Part print with two shaded views. Sizes in mm from the minimum x, y, z corner. A direction names the side the tool comes from. Give positions to 0.01 mm unless a question says otherwise; leave off trailing zeros. Order: outer loops, then holes, each group sorted by start corner. A loop starts at its lowest first (then second) coordinate and runs counter-clockwise, first axis right, second up. Notation, with made-up numbers: M 85.5,62.5 L 99.5,62.5 A26 ccw 99.5,99.5 Z; hole C 14.5,77 d11. An arc over 180 degrees is marked long. Return JSON: item names as keys, results as strings.
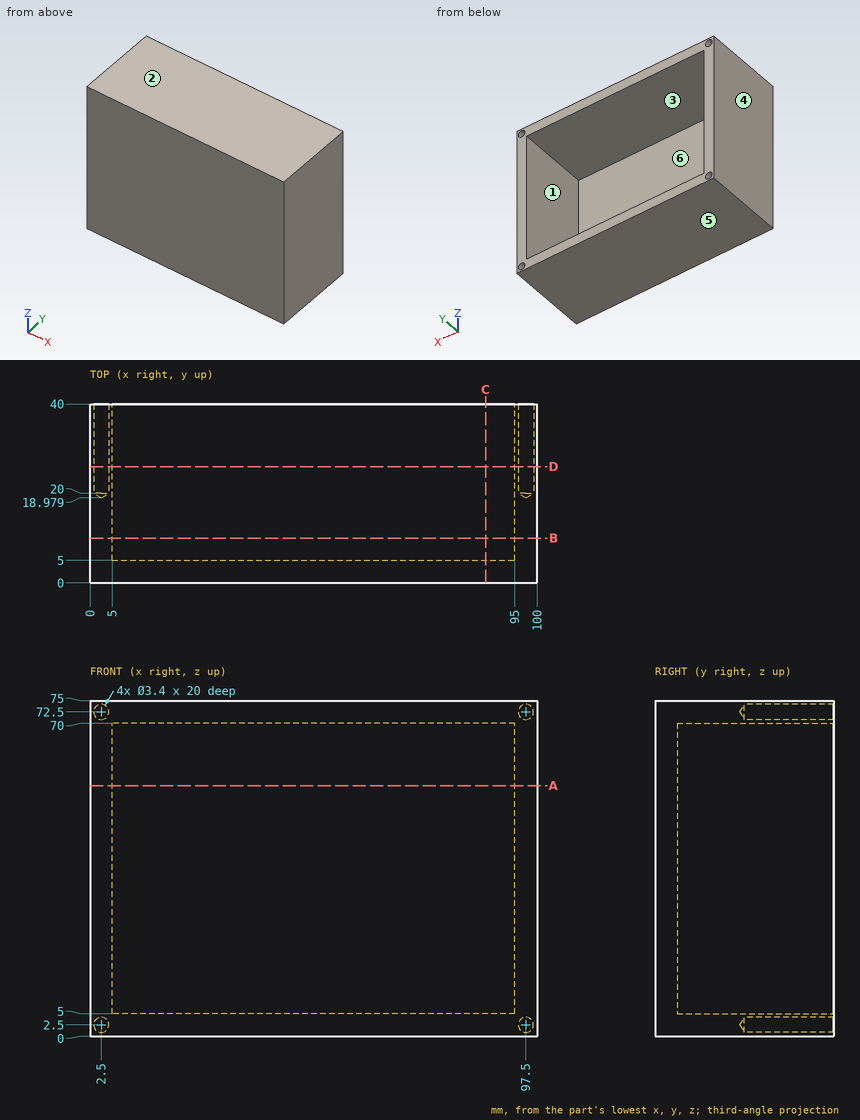
Q1. Two-plate mould, pull along Z, no slides. Class the marked faces 3, 4, 5 and 6: +Z half, -Z half, draft (parallel to the pull), parting line (faces both ways), or undercut.
Established:
{"face 3": "undercut", "face 4": "draft", "face 5": "-Z half", "face 6": "undercut"}
Q2. Band-saw the part on D-D (y = 26). Give the cut face in (x, z), then the cut area to 3 significant figures.
Established:
{"outline": "M 0,0 L 100,0 L 100,75 L 0,75 Z; hole C 2.5,2.5 d3.4; hole C 2.5,72.5 d3.4; hole M 5,5 L 95,5 L 95,70 L 5,70 Z; hole C 97.5,2.5 d3.4; hole C 97.5,72.5 d3.4", "area": "1,610 mm²"}
Q3. 3-axis set-ups, long thin cutter, end or side, ignore diameter. For the marked faces 1 and 2: which of +Z, -Z, +X, -X, +Y, -Y reach the whole face in a straight line?
Established:
{"face 1": "+Y", "face 2": "+Z, +X, -X, +Y, -Y"}
Q4. Band-saw the part on C-C (x = 88.5). Give the cut face in (y, z), then the cut area to 3 significant figures.
Established:
{"outline": "M 0,0 L 40,0 L 40,5 L 5,5 L 5,70 L 40,70 L 40,75 L 0,75 Z", "area": "725 mm²"}
Q5. Pin check, flat tips, straight feed: pin 1 (2 mm diameter, centred on x = 53.5, z = 64, fed in from +Y); pin 2 (3 mm diameter, centred on x = 2.5, z = 2.5, fed in from +Y). Stop position of each tip, or through.
Established:
{"pin 1": "stops at y = 5", "pin 2": "stops at y = 19.88"}
Q6. Probe line 1 along X through (y, z) = (33.75, 2.5); line 2 along Z through (x, y) = (97.5, 27); line 3 along X through (y, z) = (23, 45). List the from-to ranges inside material, lowest first.
Established:
{"line 1": "x = 0 to 0.8, 4.2 to 95.8, 99.2 to 100", "line 2": "z = 0 to 0.8, 4.2 to 70.8, 74.2 to 75", "line 3": "x = 0 to 5, 95 to 100"}
Q7. Band-saw the part on B-B (y = 10). Give the cut face in (x, z).
Established:
{"outline": "M 0,0 L 100,0 L 100,75 L 0,75 Z; hole M 5,5 L 95,5 L 95,70 L 5,70 Z"}
Q8. Band-saw the part on A-A (z = 56). Give the cut face in (x, y), then the cut area to 3 significant figures.
Established:
{"outline": "M 0,0 L 100,0 L 100,40 L 95,40 L 95,5 L 5,5 L 5,40 L 0,40 Z", "area": "850 mm²"}
